Geometry: see drawing. Coordinates: mm, zero at the bounding-box minimum. Coordinates: 2 decimals unless noted, no trailing zeros. Order: outer loops, then holes, each group sorted by start corner. A loop starts at its lowest first (then second) coordinate and runs counter-clockwise, first axis right, second up.
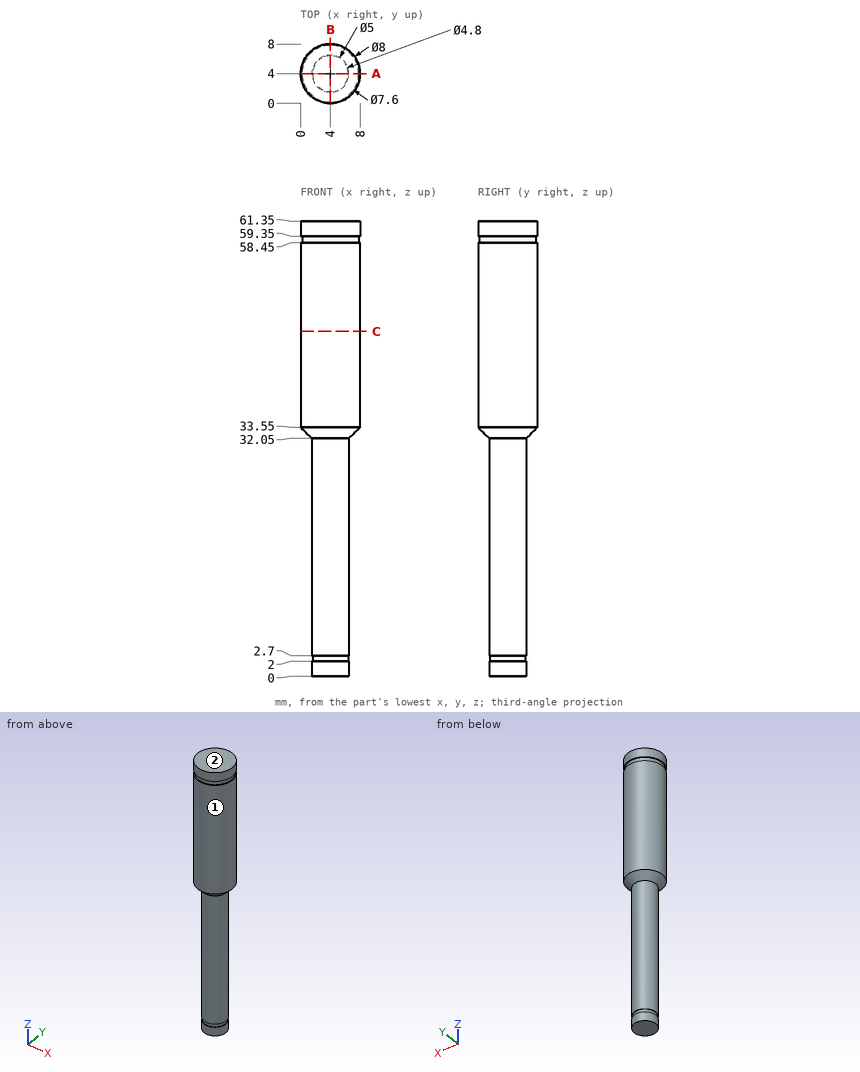
Item 1: Draft query along X for the marked faces 1 and 2. Return one class per face: pulls with the +X half, pulls with the -X half, needs draft (parallel to the pull), parting line crosses it, or undercut.
Response values:
face 1: parting line crosses it
face 2: needs draft
Item 2: Ray query, probe 1 along Y at (x, z) = (4, 26); probe 2 along Y at (x, z) = (5.75, 29); probe 3 along X at (y, z) = (5.25, 5.5). Return the intervals inside material, ascending.
Response values:
probe 1: y = 1.5 to 6.5
probe 2: y = 2.21 to 5.79
probe 3: x = 1.83 to 6.17
Item 3: Pin query (flat end, axial travel): pin 1 Ø3 at (y, z) = (4, 31.5) entering from -X; pin 2 Ø4 at (x, y) = (6.5, 4.5) entering from -Z; pin 3 Ø2 at (y, z) = (6.5, 13.5) entering from +X. Return the tip coordinate at first contact, or that it passes through.
Response values:
pin 1: stops at x = 0.55
pin 2: stops at z = 0
pin 3: stops at x = 6
Item 4: Cut plane C-C on z = 46.5. Return loops of the section in (x, y), then the cut area to 3 significant figures.
Response values:
outline: circle Ø8 at (4, 4)
area: 50.3 mm2
Item 5: Cut plane A-A on y = 4. Return loops of the section in (x, z).
Response values:
outline: (0, 33.55) - (1.5, 32.05) - (1.5, 2.7) - (1.6, 2.7) - (1.6, 2) - (1.5, 2) - (1.5, 0) - (6.5, 0) - (6.5, 2) - (6.4, 2) - (6.4, 2.7) - (6.5, 2.7) - (6.5, 32.05) - (8, 33.55) - (8, 58.45) - (7.8, 58.45) - (7.8, 59.35) - (8, 59.35) - (8, 61.35) - (0, 61.35) - (0, 59.35) - (0.2, 59.35) - (0.2, 58.45) - (0, 58.45) - close
